```python
from build123d import *

# Parameters (mm, degrees)
F2_W      = 120
F2_H      = 6
F5_D      = 12
F7_DEPTH  = 332
F9_DEPTH  = 15
F11_DEPTH = 3
F12_R     = 5
F14_D     = 35
F15_D     = 15
F16_W     = 200
F16_H     = 6
F17_DEPTH = 200
F18_DEPTH = 6
F19_W     = 60
F19_H     = 6
F19_H_2   = 226.75
F20_DEPTH = 6
F22_DEPTH = 6


# Not quite as in the source:
# - a pattern or mirror of a feature is missing from the dataset's text; its kind, count and spacing are read off the source's solid


with BuildPart() as f3:
    # F3: sweep along a path in F0
    with BuildLine(Plane.YZ) as f3_path:
        Line((-160, 150), (-160, -150))
        Line((-160, -150), (160, -150))
        Line((160, -150), (160, 150))
    # F2 (on offset) → F3 (sweep)
    with BuildSketch(Plane.XY.offset(150)):
        with Locations((0, -163)):
            Rectangle(F2_W, F2_H)
    sweep(path=f3_path.line, transition=Transition.RIGHT)

    # F5 (through all)
    with Locations(Plane.XZ.offset(166)):
        with Locations((-46, 137.25), (-46, 45.25), (46, 45.25), (46, 137.25)):
            Hole(F5_D / 2)

    # F6 (on face) → F7 (cut, through all)
    with BuildSketch(Plane.XZ.offset(166)):
        with BuildLine():
            Line((25, 150), (-25, 150))
            Line((-25, 150), (-25, 91.25))
            ThreePointArc((-25, 91.25), (0, 66.25), (25, 91.25))
            Line((25, 91.25), (25, 150))
        make_face()
    extrude(amount=-F7_DEPTH, mode=Mode.SUBTRACT)

    # F8 (on Right) → F9 (join, symmetric)
    with BuildSketch(Plane.YZ):
        Polygon((160, -150), (160, -120), (100, -150), align=None)
    f9 = extrude(amount=F9_DEPTH, both=True)

    # F9_copies: F9 across plane
    add(f9.mirror(Plane(origin=(0, 0, 0), x_dir=(0, 0, -1), z_dir=(0, -1, 0))))

    # F10 (on face) → F11 (cut)
    with BuildSketch(Plane.YZ.offset(15)):
        Polygon((116.94427191, -146), (156, -146), (156, -126.472135955), align=None)
    f11 = extrude(amount=-F11_DEPTH, mode=Mode.SUBTRACT)

    # F11_copies: F11 across plane
    add(f11.mirror(Plane(origin=(0, 0, 0), x_dir=(0, 0, -1), z_dir=(-1, 0, 0))), mode=Mode.SUBTRACT)

    # F11_copies1: F11 across plane
    add(f11.mirror(Plane(origin=(0, 0, 0), x_dir=(0, 0, -1), z_dir=(0, -1, 0))), mode=Mode.SUBTRACT)

    # F12
    f12_edges = [f3.edges().sort_by_distance(p)[0] for p in [
        (60, -163, 150),
        (-60, -163, 150),
        (-60, 163, 150),
        (60, 163, 150),
    ]]
    fillet(f12_edges, radius=F12_R)

    # F14 (through all)
    with Locations(Plane.XY.offset(-150)):
        with Locations((0, 50), (0, -50)):
            Hole(F14_D / 2)

    # F15 (through all)
    with Locations(Plane.XY.offset(-150)):
        with Locations((0, 0)):
            Hole(F15_D / 2)

    # F16 (on face) → F17 (join)
    with BuildSketch(Plane.YZ.offset(60)):
        with Locations((266, 7)):
            Rectangle(F16_W, F16_H)
    extrude(amount=-F17_DEPTH)

    # F16 (on face) → F18 (join)
    with BuildSketch(Plane.YZ.offset(60)):
        Polygon((366, 4), (166, 4), (166, -81), align=None)
    f18 = extrude(amount=-F18_DEPTH)

    # F18_copies: F18 across plane
    add(f18.mirror(Plane(origin=(0, 0, 0), x_dir=(0, 0, -1), z_dir=(-1, 0, 0))))

    # F19 (on face) → F20 (join)
    with BuildSketch(Plane.XZ.offset(-166)):
        with Locations((-110, 7)):
            Rectangle(F19_W, F19_H)
        with Locations((-110, -109.375)):
            Rectangle(F19_W, F19_H_2)
        with BuildLine():
            ThreePointArc((-131, -142.75), (-125, -136.75), (-119, -142.75))
            Line((-119, -142.75), (-119, -197.75))
            ThreePointArc((-119, -197.75), (-125, -203.75), (-131, -197.75))
            Line((-131, -197.75), (-131, -142.75))
        make_face(mode=Mode.SUBTRACT)
        with BuildLine():
            Line((-101, -197.75), (-101, -142.75))
            ThreePointArc((-101, -142.75), (-95, -136.75), (-89, -142.75))
            Line((-89, -142.75), (-89, -197.75))
            ThreePointArc((-89, -197.75), (-95, -203.75), (-101, -197.75))
        make_face(mode=Mode.SUBTRACT)
    extrude(amount=F20_DEPTH)

    # F21 (on face) → F22 (join)
    with BuildSketch(Plane(origin=(-140, 0, 0), x_dir=(0, -1, 0), z_dir=(-1, 0, 0))):
        Polygon((-166, -81), (-166, 4), (-366, 4), align=None)
    extrude(amount=-F22_DEPTH)


solid = f3.part
```
Input: part model. Units: mm. Frame: model coordinates. A direction names the side the tool comes from. Give positions to 0.01 mm unless a question says otherwise; leave off trailing zeros. Loops run counter-clockwise (first coordinate to the right, second up) from the corner with the lowest first, then second, coordinate; pieces in that order, holes last. Notation, with made-up numbers: M 31,38.5 L 46,38.5 A29 cw 46,75.5 Z; hole C 56,12 d7. An arc over 180 degrees is marked long. Answer as CSV lines item,"result". Start each with the question number.
1. Pin query (flat end, axial travel): P1, Ø3, axis at x = -74, y = 220, coming from the +Z side; P2, Ø2.5, axis at x = 13, y = 136.5, coming from the +Z side (3 decimals); P3, Ø5, axis at x = -88, y = 297.5, coming from the -Z side; P4, Ø19, axis at x = -46, z = 45.25, coming from the -Y side. Return the tip coordinate at first contact, or that it passes through.
2. Section D-D on y = 50. Return loops of the section in (x, z), plus the area to 3 significant figures.
3. Pull-direction query (X, two-part tool) for faces 1 (the face through (47.301, 163.042, 131.393)), 2 (the face through (0, 130, -135)), 3 (the face through (12, 145, -140)); classes: released by +X, released by -X, zero draft, split by the parting line, or undercut.
4. Line query: L1, parallel to Z at x = -46, y = 161.35; L2, parallel to Y at x = 33.5, z = 130; L3, parallel to Z at x = -49, y = 23. Output: solid intervals per line, ascending.
5. Section C-C on z = 45.25. Return loops of the section in (x, y).
6. Section B-B on x = 0. Return loops of the section in (y, z).
7. Reachability of faces 4 (the face through (15, 136.5, -136)), 5 (the face through (-54, 242, -28)), 6 (the face through (-1, 166, 65)), 7 (the face through (12, -145, -140)) from +Z, -Z, +X, -X, +Y, -Y: full face, straight path, thin tool, end or side. Return the list, or none.
8. Section A-A on x = -95. Return loops of the section in (y, z).
Computed values:
1,P1,"stops at z = 10"
1,P2,"stops at z = -131.125"
1,P3,"stops at z = 4"
1,P4,"stops at y = -166"
2,outline,"M -60,-156 L -17.5,-156 L -17.5,-150 L -60,-150 Z; M 17.5,-156 L 60,-156 L 60,-150 L 17.5,-150 Z"
2,area,"510 mm²"
3,face 1,"undercut"
3,face 2,"zero draft"
3,face 3,"released by +X"
4,L1,"z = -156 to 39.25, 51.25 to 131.25, 143.25 to 150"
4,L2,"y = -166 to -160, 160 to 166"
4,L3,"z = -156 to -150"
5,outline,"M -60,-166 L -52,-166 L -52,-160 L -60,-160 Z; M -60,160 L -52,160 L -52,166 L -60,166 Z; M -40,-166 L 40,-166 L 40,-160 L -40,-160 Z; M -40,160 L 40,160 L 40,166 L -40,166 Z; M 52,-166 L 60,-166 L 60,-160 L 52,-160 Z; M 52,160 L 60,160 L 60,166 L 52,166 Z"
6,outline,"M -166,-156 L -67.5,-156 L -67.5,-150 L -100,-150 L -160,-120 L -160,66.25 L -166,66.25 Z; M -32.5,-156 L -7.5,-156 L -7.5,-150 L -32.5,-150 Z; M 7.5,-156 L 32.5,-156 L 32.5,-150 L 7.5,-150 Z; M 67.5,-156 L 166,-156 L 166,4 L 366,4 L 366,10 L 166,10 L 166,66.25 L 160,66.25 L 160,-120 L 100,-150 L 67.5,-150 Z"
7,face 4,"+Z, +X"
7,face 5,"-Z, +Y"
7,face 6,"+Z, +X, -X, +Y"
7,face 7,"+X"
8,outline,"M 160,-222.75 L 166,-222.75 L 166,-203.75 L 160,-203.75 Z; M 160,-136.75 L 166,-136.75 L 166,4 L 366,4 L 366,10 L 160,10 Z"
